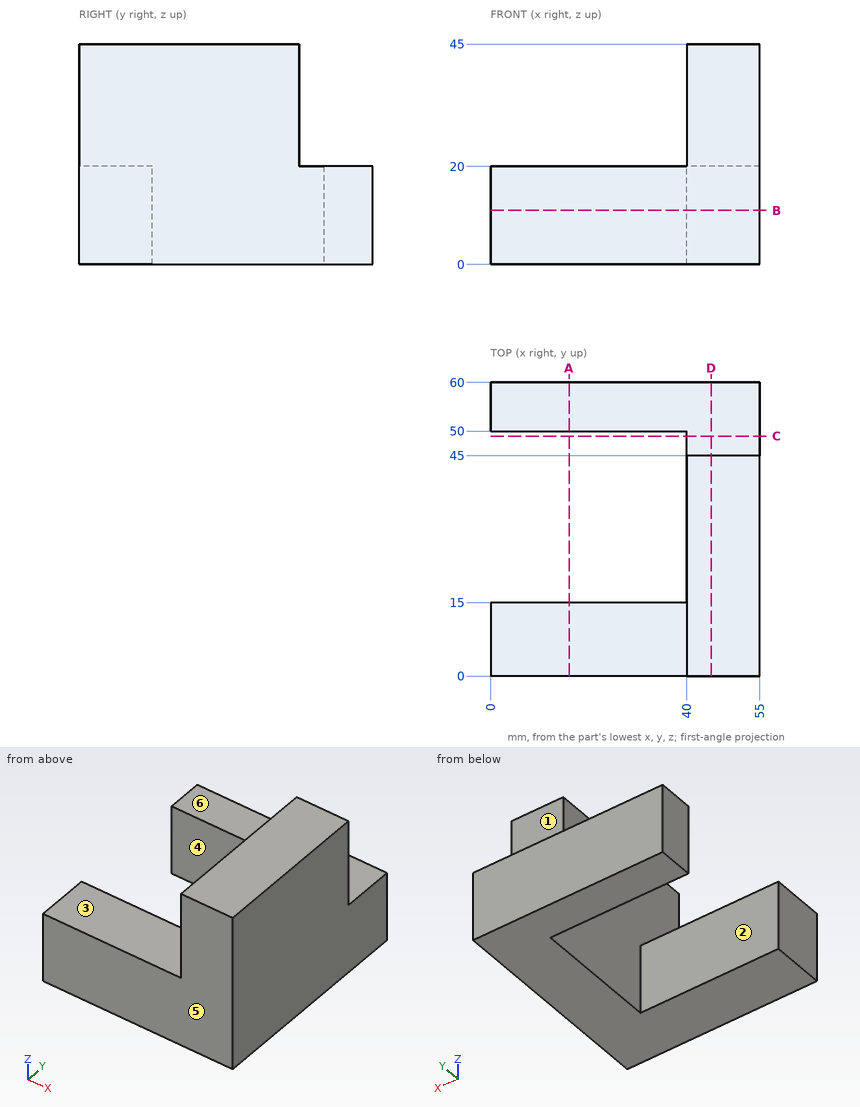
Print and shaded views of the part. All mm, measured from the part's lowest x, y and z. A direction names the side the tool comes from. Coordinates: 2 decimals unless noted, no trailing zeros. Loops run counter-clockwise (first coordinate to the right, second up) from the corner with the lowest first, then second, coordinate; pieces in that order, holes last. Notation, with made-up numbers: (-5.5, 5.25) - (32.5, 5.25) arc R23 cw to (32.5, 37.25) - close; hole circle Ø5 at (17.25, 79). An arc over 180 degrees is marked (long way). Use one line per item in the form item = value. Start each with the question number.
1) Band-saw the part on C-C (y = 49). Give the cut face in (x, z).
2) Band-saw the part on B-B (z = 11). Give the cut face in (x, y).
3) Tool access for the marked faces 4, 5 and 6: list every direction of +Z, -Z, +X, -X, +Y, -Y with a clear straight run to the whole face (end or side of a thin tool).
4) Band-saw the part on D-D (x = 45). Give the cut face in (y, z).
5) Drill centre lines: L1, parallel to Y at x = 19.5, z = 7; L2, parallel to X at y = 27.5, z = 13; L3, parallel to Z at x = 29, y = 7. Where is each one in solid material? Low to high. Write a range as from..to.
6) Flat gauge pins, fed straight in: pin 1 (10 mm diameter, centred on y = 13.5, z = 39.5, fed in from -X); pin 2 (12 mm diameter, centred on x = 47.5, z = 29, fed in from +Y); pin 3 (7.5 mm diameter, centred on x = 17.5, y = 52.5, fed in from +Z). Where does each tip first touch, or does it go through?
7) Two-plate mould, pull along Y, no slides. Class the marked faces 1, 2 and 3: +Y half, -Y half, draft (parallel to the pull), parting line (faces both ways), or undercut.
8) Band-saw the part on A-A (x = 16). Give the cut face in (y, z), and give its area (3 significant figures).
Check values:
q1.outline = (40, 0) - (55, 0) - (55, 20) - (40, 20) - close
q2.outline = (0, 0) - (55, 0) - (55, 60) - (0, 60) - (0, 50) - (40, 50) - (40, 15) - (0, 15) - close
q3.face_4 = +Z, -Z, -X
q3.face_5 = +Z, -Z, +X, -X, -Y
q3.face_6 = +Z, +X, -X, +Y
q4.outline = (0, 0) - (60, 0) - (60, 20) - (45, 20) - (45, 45) - (0, 45) - close
q5.L1 = 0..15, 50..60
q5.L2 = 40..55
q5.L3 = 0..20
q6.pin_1 = 40
q6.pin_2 = 45
q6.pin_3 = 20
q7.face_1 = +Y half
q7.face_2 = undercut
q7.face_3 = draft
q8.outline = (0, 0) - (15, 0) - (15, 20) - (0, 20) - close; (50, 0) - (60, 0) - (60, 20) - (50, 20) - close
q8.area = 500 mm2
